Part model, mm, in its own coordinate system. A direction names the side the tool comes from. Round coordinates to 2 decimals unless told otherwise and drop trailing zeros. Write each loop counter-clockwise with the first axis right and the second up, starting at its lowest first coordinate (ties: lowest second). Pieces come first, ordered by that corner, then holes. Notation, with made-up numbers: M 89,10.25 L 124,10.25 A25 cw 124,23.25 Z; hole C 44.25,-17 d2. An arc over 180 degrees is marked long. Use one line per item in the form item = value. Start each with the question number.
Item 1: Which spindle directions (+Z, -Z, +X, -X, +Y, -Y) get a long thin tool onto all of the face, cutting with end or side? Do faces 1 (the face through (0.142, -16, 8)), 2 (the face through (-12, -13, 5)), 3 (the face through (-17, 2.454, 9)), 4 (the face through (-17, -2.546, 9)), 5 (the face through (14.29, -14.14, 7.54)). Say none if no direction does.
Item 2: Probe L1, parallel to Z at x = 12.5, y = -11.5; L2, parallel to Y at x = 0, z = 4.5; L3, parallel to X at y = 0.5, z = 6.5 (1 decimal). List the from-to ranges inside material, lowest first.
Item 3: Cut at D-D, the plane y = 11. Give the cut face in (x, z).
Item 4: Flat gauge pins, fed straight in: pin 1 Ø2 at (y, z) = (-8.5, 5.5) entering from -X; pin 2 Ø4 at (x, y) = (1, 9) entering from -Z; pin 3 Ø1.5 at (x, z) = (17.5, 6.5) entering from -Y; pin 4 Ø0.9 at (y, z) = (-15.5, 8.5) entering from -X. Where does each tip first touch, or does it go through?
Item 5: Cut at C-C, the plane y = -7. State how many separate pieces and enclosed holes the cut face has, then the cut area to 3 significant figures.
Item 6: Mould opens along Y. For faces 6 (the face through (12, -12.39, 5.96)), 7 (the face through (16, -7, 5)), 8 (the face through (-14.662, -8.696, 8.091)), 9 (the face through (-14.246, -14.196, 7.535)) say: +Y half, -Y half, draft (parallel to the pull), parting line (faces both ways), or undercut.
Item 7: Cut at B-B, the plane z = 0.5. Give the cut face in (x, y).
Item 8: Cut at A-A, the plane y = 0. Give the cut face in (x, z), then the cut area to 3 significant figures.
from build123d import *

# Parameters (mm, degrees)
ESQUISSE1_R             = 15
ESQUISSE1_R_2           = 10
BOSS_EXTRU_1_DEPTH      = 10
ESQUISSE2_W             = 7
ESQUISSE2_H             = 5
ESQUISSE2_W_2           = 0.284758048
ESQUISSE2_H_2           = 1.526135502
BOSS_EXTRU_2_DEPTH      = 5
ESQUISSE3_R             = 1
ENL_V_MAT_EXTRU_1_DEPTH = 10
ESQUISSE4_R             = 1
ENL_V_MAT_EXTRU_2_DEPTH = 7
ESQUISSE5_R             = 1
ENL_V_MAT_EXTRU_3_DEPTH = 7


with BuildPart() as part:
    # Esquisse1 → Boss.-Extru.1 (new body)
    with BuildSketch(Plane.XY):
        Circle(ESQUISSE1_R)
        Circle(ESQUISSE1_R_2, mode=Mode.SUBTRACT)
    extrude(amount=BOSS_EXTRU_1_DEPTH)

    # Esquisse2 → Boss.-Extru.2 (add)
    with BuildSketch(Plane.XY.offset(10)):
        with Locations((-16.5, -0.045599179)):
            Rectangle(ESQUISSE2_W, ESQUISSE2_H)
        Polygon((-12.723746603, -2.860261308), (-11.24279347, -7.635905538), (-17.928695393, -9.709239924), (-19.409648526, -4.933595693), align=None)
        Polygon((-10.38626352, -7.829614824), (-7.248762671, -11.722696948), (-12.699077643, -16.115198137), (-15.836578493, -12.222116013), align=None)
        Polygon((15.836578493, -12.222116013), (12.699077643, -16.115198137), (7.248762671, -11.722696948), (10.38626352, -7.829614824), align=None)
        Polygon((19.409648526, -4.933595693), (17.928695393, -9.709239924), (11.24279347, -7.635905538), (12.723746603, -2.860261308), align=None)
        with Locations((16.5, -0.045599179)):
            Rectangle(ESQUISSE2_W, ESQUISSE2_H)
        with Locations((0, -15.401311239)):
            Rectangle(ESQUISSE2_W_2, ESQUISSE2_H_2)
    extrude(amount=-BOSS_EXTRU_2_DEPTH)

    # Esquisse3 → Enlèv. mat.-Extru.1 (cut)
    with BuildSketch(Plane.XZ.offset(2.545599179)):
        with Locations((-17.292317554, 7.389299581)):
            Circle(ESQUISSE3_R)
    enl_v_mat_extru_1 = extrude(amount=-ENL_V_MAT_EXTRU_1_DEPTH, mode=Mode.SUBTRACT)

    # Esquisse4 → Enlèv. mat.-Extru.2 (cut)
    with BuildSketch(Plane(origin=(1.17388153, -3.785427393, 0), x_dir=(0.955128846150379, 0.2961906265421742, 0), z_dir=(0.2961906265421742, -0.955128846150379, 0))):
        with Locations((-17.565905228, 7.267460252)):
            Circle(ESQUISSE4_R)
    enl_v_mat_extru_2 = extrude(amount=-ENL_V_MAT_EXTRU_2_DEPTH, mode=Mode.SUBTRACT)

    # Esquisse5 → Enlèv. mat.-Extru.3 (cut)
    with BuildSketch(Plane(origin=(2.873250851, -3.56519474, 0), x_dir=(0.778616424708494, 0.6275001698598672, 0), z_dir=(0.6275001698598671, -0.7786164247084939, 0))):
        with Locations((-16.898350616, 6.935079558)):
            Circle(ESQUISSE5_R)
    enl_v_mat_extru_3 = extrude(amount=-ENL_V_MAT_EXTRU_3_DEPTH, mode=Mode.SUBTRACT)

    # Symétrie1: Enlèv. mat.-Extru.1, Enlèv. mat.-Extru.2, Enlèv. mat.-Extru.3 across plane
    add(enl_v_mat_extru_1.mirror(Plane(origin=(0, 0, 0), x_dir=(0, 0, 1), z_dir=(1, 0, 0))), mode=Mode.SUBTRACT)
    add(enl_v_mat_extru_2.mirror(Plane(origin=(0, 0, 0), x_dir=(0, 0, 1), z_dir=(1, 0, 0))), mode=Mode.SUBTRACT)
    add(enl_v_mat_extru_3.mirror(Plane(origin=(0, 0, 0), x_dir=(0, 0, 1), z_dir=(1, 0, 0))), mode=Mode.SUBTRACT)


solid = part.part
Model answer:
q1.face_1 = +Z, -Z, -Y
q1.face_2 = -Z, -X, -Y
q1.face_3 = +Z, -Z, -X, +Y
q1.face_4 = +Z, -Z, -X
q1.face_5 = +Z, -Z, +X, -Y
q2.L1 = 5 to 5.94, 7.93 to 10
q2.L2 = -15 to -10, 10 to 15
q2.L3 = -20 to -17.7, -16.8 to -10, 10 to 16.8, 17.7 to 20
q3.outline = M -10.2,0 L 10.2,0 L 10.2,10 L -10.2,10 Z
q4.pin_1 = -18.61
q4.pin_2 = 0
q4.pin_3 = -9.71
q4.pin_4 = -13.56
q5.separate_pieces = 2
q5.enclosed_holes = 2
q5.area = 171 mm²
q6.face_6 = undercut
q6.face_7 = draft
q6.face_8 = undercut
q6.face_9 = -Y half
q7.outline = C 0,0 d30; hole C 0,0 d20
q8.outline = M -20,5 L -15,5 L -15,0 L -10,0 L -10,10 L -20,10 Z; M 10,0 L 15,0 L 15,5 L 20,5 L 20,10 L 10,10 Z; hole C -17.29,7.39 d2; hole C 17.29,7.39 d2
q8.area = 144 mm²
